Can you work these out from the model? Positions are in its coordinate system, mm. Face numbers are marked on the shaded views. Give positions to 0.01 mm unless a question says otherwise; leave off trailing zeros. Write each loop counter-clockwise with the first axis right and the second up, starting at its lowest first coordinate (ties: lowest second). Pieces come first, ordered by that corner, then holes.
1. I'm going to push flat-ended pins straight in: pin 1 (8 mm diameter, centred on x = -5, z = 1.5, fed in from +Y); pin 2 (1.2 mm diameter, centred on x = 4, z = -10.25, fed in from -Y). Where does each tip first touch, or does it pass through?
2. Thinking about a two-plate mould opening in X: for the marked faces 1, 2 and 3, which applies, pulls with the +X half, pulls with the -X half, needs draft (parallel to the pull), parting line crosses it, or undercut?
3. Suppose I cut it at C-C (z = -10.25). Please give me the cut outline in (x, y), and give its area (3 significant figures).
4. If I drill on probe 1 along X at (y, z) = (-1.2, -10.25); probe 2 along Y at (x, z) = (6.75, -11); probe 3 along Z at (x, y) = (-9.75, 4), over which ranges is the centre line in solid material (lowest first)?
5. Suppose I cut it at A-A (x = -4). Please give me the cut outline in (y, z).
6. Suppose I cut it at B-B (y = 4). Please give me the cut outline in (x, z), and give its area (3 significant figures).
7. Suppose I cut it at D-D (z = 9.5). Please give me the cut outline in (x, y).
```python
from build123d import *

# Parameters (mm, degrees)
SKETCH1_R             = 1.25
BOSS_EXTRUDE1_DEPTH   = 10
BOSS_EXTRUDE1_2_DEPTH = 10
BOSS_EXTRUDE1_3_DEPTH = 10
BOSS_EXTRUDE1_4_DEPTH = 10
SKETCH2_W             = 26.5
SKETCH2_H             = 26.5
BOSS_EXTRUDE2_DEPTH   = 2
SKETCH3_R             = 1
CUT_EXTRUDE1_DEPTH    = 1.5


with BuildPart() as part:
    # Sketch1 → Boss-Extrude1 (new body)
    with BuildSketch(Plane(origin=(0, 0, 0), x_dir=(1, 0, 0), z_dir=(0, 1, 0))):
        with Locations(Location((-10.25, -10.25, 0), (0, 0, 270))):
            Circle(SKETCH1_R)
    extrude(amount=BOSS_EXTRUDE1_DEPTH)



with BuildPart() as body_2:
    # Sketch1 → Boss-Extrude1 2 (new body)
    with BuildSketch(Plane(origin=(0, 0, 0), x_dir=(1, 0, 0), z_dir=(0, 1, 0))):
        with Locations(Location((-10.25, 10.25, 0), (0, 0, 270))):
            Circle(SKETCH1_R)
    extrude(amount=BOSS_EXTRUDE1_2_DEPTH)


with BuildPart() as body_3:
    # Sketch1 → Boss-Extrude1 3 (new body)
    with BuildSketch(Plane(origin=(0, 0, 0), x_dir=(1, 0, 0), z_dir=(0, 1, 0))):
        with Locations(Location((10.25, 10.25, 0), (0, 0, 270))):
            Circle(SKETCH1_R)
    extrude(amount=BOSS_EXTRUDE1_3_DEPTH)


with BuildPart() as body_4:
    # Sketch1 → Boss-Extrude1 4 (new body)
    with BuildSketch(Plane(origin=(0, 0, 0), x_dir=(1, 0, 0), z_dir=(0, 1, 0))):
        with Locations(Location((10.25, -10.25, 0), (0, 0, 270))):
            Circle(SKETCH1_R)
    extrude(amount=BOSS_EXTRUDE1_4_DEPTH)


with BuildPart() as part_1:
    add(part.part)

    add(body_2.part)  # Boss-Extrude2 merges body 2

    add(body_3.part)  # Boss-Extrude2 merges body 3

    add(body_4.part)  # Boss-Extrude2 merges body 4
    # Sketch2 → Boss-Extrude2 (add)
    with BuildSketch(Plane.XZ):
        Rectangle(SKETCH2_W, SKETCH2_H)
    extrude(amount=BOSS_EXTRUDE2_DEPTH)

    # Sketch3 → Cut-Extrude1 (cut)
    with BuildSketch(Plane.XZ.offset(2)):
        with Locations(Location((-4, -10.25, 0), (0, 0, 270))):
            Circle(SKETCH3_R)
        with Locations(Location((4, -10.25, 0), (0, 0, 270))):
            Circle(SKETCH3_R)
    extrude(amount=-CUT_EXTRUDE1_DEPTH, mode=Mode.SUBTRACT)


solid = part_1.part
```
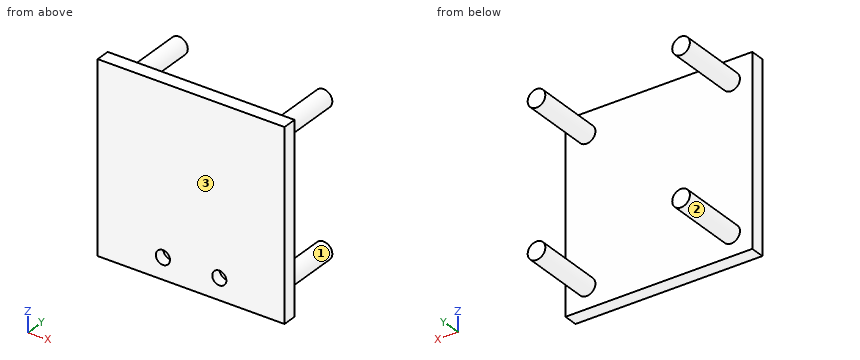
Checks:
1. pin 1: stops at y = 0
1. pin 2: stops at y = -0.5
2. face 1: undercut
2. face 2: undercut
2. face 3: needs draft
3. outline: (-13.25, -2) - (-5, -2) - (-5, -0.5) - (-3, -0.5) - (-3, -2) - (3, -2) - (3, -0.5) - (5, -0.5) - (5, -2) - (13.25, -2) - (13.25, 0) - (11.5, 0) - (11.5, 10) - (9, 10) - (9, 0) - (-9, 0) - (-9, 10) - (-11.5, 10) - (-11.5, 0) - (-13.25, 0) - close
3. area: 97.0 mm2
4. probe 1: x = -13.25 to -5, -3 to 3, 5 to 13.25
4. probe 2: y = -2 to 0
4. probe 3: z = -11.4 to -9.1, 9.1 to 11.4
5. outline: (-2, -13.25) - (0, -13.25) - (0, 13.25) - (-2, 13.25) - (-2, -9.25) - (-0.5, -9.25) - (-0.5, -11.25) - (-2, -11.25) - close
6. outline: circle Ø2.5 at (-10.25, -10.25); circle Ø2.5 at (-10.25, 10.25); circle Ø2.5 at (10.25, -10.25); circle Ø2.5 at (10.25, 10.25)
6. area: 19.6 mm2
7. outline: (-13.25, -2) - (13.25, -2) - (13.25, 0) - (11.25, 0) - (11.25, 10) - (9.25, 10) - (9.25, 0) - (-9.25, 0) - (-9.25, 10) - (-11.25, 10) - (-11.25, 0) - (-13.25, 0) - close
